from build123d import *

# Parameters (mm, degrees)
SKETCH2_R         = 2.413
EXTRUDE1_DEPTH    = 9.525
CHAMFER1_SIZE     = 0.5953125
EXTRUDE4_DEPTH    = 9.525
SKETCH8_OUTSIDE_W = 85.776
SKETCH8_OUTSIDE_H = 87.248
SKETCH8_OUTSIDE_R = 4.7625
EXTRUDE5_DEPTH    = 20.05
EXTRUDE5_TAPER    = 60
SKETCH9_OUTSIDE_W = 52.78
SKETCH9_OUTSIDE_H = 54.252
SKETCH9_OUTSIDE_R = 4.7625
EXTRUDE6_DEPTH    = 10.525
EXTRUDE6_TAPER    = 60
SKETCH10_R        = 2.413
EXTRUDE7_DEPTH    = 4.7625


with BuildPart() as part:
    # Sketch2 → Extrude1 (new body)
    with BuildSketch(Plane(origin=(9.525, 0, 0), x_dir=(0, 0, -1), z_dir=(1, 0, 0))):
        Circle(SKETCH2_R)
    extrude(amount=-EXTRUDE1_DEPTH)

    # Chamfer1
    chamfer1_edges = [part.edges().sort_by_distance(p)[0] for p in [
        (9.525, 0, 2.413),
    ]]
    chamfer(chamfer1_edges, length=CHAMFER1_SIZE)

    # Sketch7 → Extrude4 (add)
    with BuildSketch(Plane(origin=(0, 0, 0), x_dir=(0, 0, -1), z_dir=(1, 0, 0))):
        Polygon((0, 5.499261314), (-4.7625, 2.749630657), (-4.7625, -2.749630657), (0, -5.499261314), (4.7625, -2.749630657), (4.7625, 2.749630657), align=None)
    extrude(amount=-EXTRUDE4_DEPTH)

    # Sketch8 outside → Extrude5 (cut, through all)
    with BuildSketch(Plane.ZY.offset(9.525)):
        Rectangle(SKETCH8_OUTSIDE_W, SKETCH8_OUTSIDE_H)
        Circle(SKETCH8_OUTSIDE_R, mode=Mode.SUBTRACT)
    extrude(amount=-EXTRUDE5_DEPTH, taper=EXTRUDE5_TAPER, mode=Mode.SUBTRACT)

    # Sketch9 outside → Extrude6 (cut, through all)
    with BuildSketch(Plane(origin=(0, 0, 0), x_dir=(0, 0, -1), z_dir=(1, 0, 0))):
        Rectangle(SKETCH9_OUTSIDE_W, SKETCH9_OUTSIDE_H)
        Circle(SKETCH9_OUTSIDE_R, mode=Mode.SUBTRACT)
    extrude(amount=-EXTRUDE6_DEPTH, taper=EXTRUDE6_TAPER, mode=Mode.SUBTRACT)

    # Sketch10 → Extrude7 (cut)
    with BuildSketch(Plane.ZY.offset(9.525)):
        Circle(SKETCH10_R)
    extrude(amount=-EXTRUDE7_DEPTH, mode=Mode.SUBTRACT)


solid = part.part
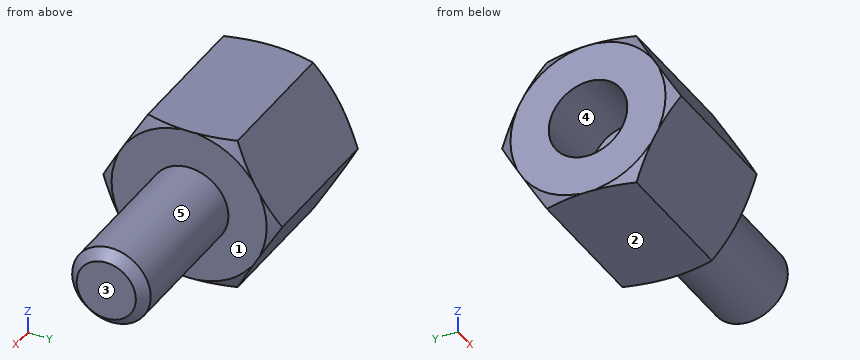
Verification items for the finished model (mm, model axes). Face numbers are marked on the shaded views. A direction names the side the tool comes from. Coordinates: 2 decimals unless noted, no trailing zeros. Loops run counter-clockwise (first coordinate to the right, second up) from the corner with the lowest first, then second, coordinate; pieces in that order, holes last. Notation, with made-up numbers: M 1.25,60.25 L 38.25,60.25 A23 ccw 38.25,99.25 Z; hole C -39.75,36.25 d3. An arc over 180 degrees is marked long. One line per item, written item: value.
1. Material ranges on line 1 along X through (y, z) = (-2.5, 2.5) (3 decimals); line 2 along Z through (x, y) = (-7.25, -2); line 3 along Y through (x, z) = (3.5, 0), recorded low to high. Write a range as from..to.
Answers follow:
line 1: -9.525..0
line 2: -4.76..-1.35, 1.35..4.76
line 3: -2.41..2.41
2. Section check A-A on x = -5.5. Record the cut outline in (y, z).
Answers follow:
outline: M -5.5,0 L -2.75,-4.76 L 2.75,-4.76 L 5.5,0 L 2.75,4.76 L -2.75,4.76 Z; hole C 0,0 d4.83
3. Section check B-B on x = 5.5. Record the cut outline in (y, z).
Answers follow:
outline: C 0,0 d4.83
4. Gauge pin test, flat ends, axial feed: P1, Ø4, axis at y = 0, z = 0, coming from the -X side; P2, Ø1, axis at x = -5.5, z = 3.5, coming from the -Y side; P3, Ø2, axis at x = 2, z = 2.5, coming from the -Y side. Record the tip position at first contact, or that the pin passes through.
Answers follow:
P1: x = -4.76
P2: y = -3.77
P3: y = -1.89
5. Set-up check for the marked faces 1 and 2: record each of +Z, -Z, +X, -X, +Y, -Y from which the full face is reachable in a straight line by a thin tool's end or side.
Answers follow:
face 1: +X
face 2: -Z, +X, -X, +Y, -Y
6. Mould release check, pull along Y, two halves, no side actions. Record for the marked faces 3, 4 and 5: pulls with the +Y half, pulls with the -Y half, needs draft (parallel to the pull), parting line crosses it, or undercut.
Answers follow:
face 3: needs draft
face 4: undercut
face 5: parting line crosses it
